Could you check a few things on this model? Use its own coordinates, in mm. A direction names the side the tool comes from. Round coordinates to 2 decimals unless told otherwise and drop trailing zeros. Loops run counter-clockwise (first coordinate to the right, second up) from the corner with the lowest first, then second, coordinate; pieces in that order, holes last. Notation, with made-up numbers: (76.5, 75) -> (94.5, 75) arc R15 ccw to (94.5, 96) -> close; hole circle Ø9 at (65, -15). An arc over 180 degrees is marked (long way). Put each result on its own line as item: value. Start each with the question number.
1. I need wall thicknesses on line 1 (X direction, y = 0, z = -9); line 2 (Z direction, x = 0.55, y = 1.5); line 3 (Y direction, x = 0.15, z = -10.75). Which ranges of each line are inside material? Lowest first, please. Write a range as [from, to].
2. Imagine slicing it at A-A, the plane z = -12.75. Please give me the cut outline in (x, y), and give its area (3 significant figures).
3. I'm going to push flat-ended pins straight in: P1, Ø1.5, axis at x = 2, z = -8, coming from the +Y side; P2, Ø1.5, axis at x = -0.5, z = -4.5, coming from the -Y side; P3, Ø1, axis at x = -1, y = 0, coming from the -Z side (3 decimals). Where does each tip first touch, or does it pass through?
4. Imagine slicing it at B-B, the plane z = -1. Please give me the cut outline in (x, y), and give its area (3 significant figures).
5. Imagine slicing it at D-D, the plane z = 1.75. Please give me the cut outline in (x, y), and give its area (3 significant figures).
6. Which directions (+Z, -Z, +X, -X, +Y, -Y) give clear straight access to the entire face, cutting with the end or side of a thin tool? Please do faces 1 (the flat face through (-1.2, -1.3, 0)), 2 (the flat face through (1.394, 2.37, -7.451)).
7. Imagine slicing it at C-C, the plane y = 2. Please give me the cut outline in (x, z).
8. If we mould it in two halves opening along Y, with no side actions, what happens to faces 3 (the cylindrical face through (-1.5, 0.07, 1.36)), 4 (the flat face through (-1.394, -2.37, -7.451)), 5 (the flat face through (2.75, 0, -7)), 6 (the cylindrical face through (-0.27, -1.22, -10.81))? For each: pulls with the +Y half, pulls with the -Y half, needs draft (parallel to the pull), parting line crosses it, or undercut.
```python
from build123d import *
from OCP.BRepFilletAPI import BRepFilletAPI_MakeChamfer

# Parameters (mm, degrees)
EXTRUDE_1_DEPTH      = 15
M3X0_5_1_D           = 2.5
M3X0_5_1_DEPTH       = 8
M3X0_5_1_CSINK_D     = 3.05
M3X0_5_1_CSINK_ANGLE = 90
M3X0_5_1_TIP         = 0.751075774
SKETCH_4_R           = 1.5
EXTRUDE_2_DEPTH      = 3
CHAMFER_1_SIZE       = 0.25
CHAMFER_2_SIZE       = 0.25
CHAMFER_2_SIZE2      = 0.144337567


with BuildPart() as part:
    # ｽｹｯﾁ1 → ﾎﾞｽ - 押し出し1 (new body)
    with BuildSketch(Plane.XY):
        Polygon((-2.75, 1.58771324), (-2.75, -1.58771324), (0, -3.175426481), (2.75, -1.58771324), (2.75, 1.58771324), (0, 3.175426481), align=None)
    extrude(amount=-EXTRUDE_1_DEPTH)

    # M3x0.5 ねじ穴1
    with Locations(Plane(origin=(0, 0, -15), x_dir=(-1, 0, 0), z_dir=(0, 0, -1))):
        with Locations((0, 0)):
            CounterSinkHole(M3X0_5_1_D / 2, M3X0_5_1_CSINK_D / 2, depth=M3X0_5_1_DEPTH, counter_sink_angle=M3X0_5_1_CSINK_ANGLE)
            with Locations((0, 0, -(M3X0_5_1_DEPTH + M3X0_5_1_TIP / 2))):  # 118° drill point
                Cone(0, M3X0_5_1_D / 2, M3X0_5_1_TIP, mode=Mode.SUBTRACT)

    # ｽｹｯﾁ4 → ﾎﾞｽ - 押し出し2 (add)
    with BuildSketch(Plane.XY):
        Circle(SKETCH_4_R)
    extrude(amount=EXTRUDE_2_DEPTH)

    # 面取り1
    chamfer_1_edges = [part.edges().sort_by_distance(p)[0] for p in [
        (-1.5, 0, 3),
    ]]
    chamfer(chamfer_1_edges, length=CHAMFER_1_SIZE)

    # 面取り2: one chamfer whose edges measure the first distance from different faces: ONE call of the kernel's chamfer builder (chamfer() names one face for all edges)
    chamfer_2_edges_1 = [part.edges().sort_by_distance(p)[0] for p in [
        (-1.375, -2.38156986, -15),
        (1.375, -2.38156986, -15),
        (2.75, 0, -15),
        (1.375, 2.38156986, -15),
        (-1.375, 2.38156986, -15),
        (-2.75, 0, -15),
    ]]
    chamfer_2_side_1 = [part.faces().sort_by_distance(p)[0] for p in [
        (-2.665986112, 0, -15),
    ]]
    chamfer_2_edges_2 = [part.edges().sort_by_distance(p)[0] for p in [
        (1.375, 2.38156986, 0),
    ]]
    chamfer_2_side_2 = [part.faces().sort_by_distance(p)[0] for p in [
        (1.375, 2.38156986, -7.5),
    ]]
    chamfer_2_edges_3 = [part.edges().sort_by_distance(p)[0] for p in [
        (2.75, 0, 0),
    ]]
    chamfer_2_side_3 = [part.faces().sort_by_distance(p)[0] for p in [
        (2.75, 0, -7.5),
    ]]
    chamfer_2_edges_4 = [part.edges().sort_by_distance(p)[0] for p in [
        (1.375, -2.38156986, 0),
    ]]
    chamfer_2_side_4 = [part.faces().sort_by_distance(p)[0] for p in [
        (1.375, -2.38156986, -7.5),
    ]]
    chamfer_2_edges_5 = [part.edges().sort_by_distance(p)[0] for p in [
        (-1.375, -2.38156986, 0),
    ]]
    chamfer_2_side_5 = [part.faces().sort_by_distance(p)[0] for p in [
        (-1.375, -2.38156986, -7.5),
    ]]
    chamfer_2_edges_6 = [part.edges().sort_by_distance(p)[0] for p in [
        (-2.75, 0, 0),
    ]]
    chamfer_2_side_6 = [part.faces().sort_by_distance(p)[0] for p in [
        (-2.75, 0, -7.5),
    ]]
    chamfer_2_edges_7 = [part.edges().sort_by_distance(p)[0] for p in [
        (-1.375, 2.38156986, 0),
    ]]
    chamfer_2_side_7 = [part.faces().sort_by_distance(p)[0] for p in [
        (-1.375, 2.38156986, -7.5),
    ]]
    chamfer_2 = BRepFilletAPI_MakeChamfer(part.part.solid().wrapped)
    for e in chamfer_2_edges_1:
        chamfer_2.Add(CHAMFER_2_SIZE, CHAMFER_2_SIZE2, e.wrapped, chamfer_2_side_1[0].wrapped)  # the first distance lies on this face
    for e in chamfer_2_edges_2:
        chamfer_2.Add(CHAMFER_2_SIZE, CHAMFER_2_SIZE2, e.wrapped, chamfer_2_side_2[0].wrapped)  # the first distance lies on this face
    for e in chamfer_2_edges_3:
        chamfer_2.Add(CHAMFER_2_SIZE, CHAMFER_2_SIZE2, e.wrapped, chamfer_2_side_3[0].wrapped)  # the first distance lies on this face
    for e in chamfer_2_edges_4:
        chamfer_2.Add(CHAMFER_2_SIZE, CHAMFER_2_SIZE2, e.wrapped, chamfer_2_side_4[0].wrapped)  # the first distance lies on this face
    for e in chamfer_2_edges_5:
        chamfer_2.Add(CHAMFER_2_SIZE, CHAMFER_2_SIZE2, e.wrapped, chamfer_2_side_5[0].wrapped)  # the first distance lies on this face
    for e in chamfer_2_edges_6:
        chamfer_2.Add(CHAMFER_2_SIZE, CHAMFER_2_SIZE2, e.wrapped, chamfer_2_side_6[0].wrapped)  # the first distance lies on this face
    for e in chamfer_2_edges_7:
        chamfer_2.Add(CHAMFER_2_SIZE, CHAMFER_2_SIZE2, e.wrapped, chamfer_2_side_7[0].wrapped)  # the first distance lies on this face
    add(Compound.cast(chamfer_2.Shape()), mode=Mode.REPLACE)


solid = part.part
```
Entries:
1. line 1: [-2.75, -1.25], [1.25, 2.75]
1. line 2: [-15, 0]
1. line 3: [-3.09, -1.24], [1.24, 3.09]
2. outline: (-2.75, -1.59) -> (0, -3.18) -> (2.75, -1.59) -> (2.75, 1.59) -> (0, 3.18) -> (-2.75, 1.59) -> close; hole circle Ø2.5 at (0, 0)
2. area: 21.3 mm^2
3. P1: y = 2.45
3. P2: y = -3.18
3. P3: z = -14.975
4. outline: (-2.75, -1.59) -> (0, -3.18) -> (2.75, -1.59) -> (2.75, 1.59) -> (0, 3.18) -> (-2.75, 1.59) -> close
4. area: 26.2 mm^2
5. outline: circle Ø3 at (0, 0)
5. area: 7.07 mm^2
6. face 1: +Z
6. face 2: +Z, -Z, +X, +Y
7. outline: (-2.04, -14.86) -> (-1.54, -15) -> (1.54, -15) -> (2.04, -14.86) -> (2.04, -0.25) -> (1.75, 0) -> (-1.75, 0) -> (-2.04, -0.25) -> close
8. face 3: parting line crosses it
8. face 4: pulls with the -Y half
8. face 5: needs draft
8. face 6: undercut
